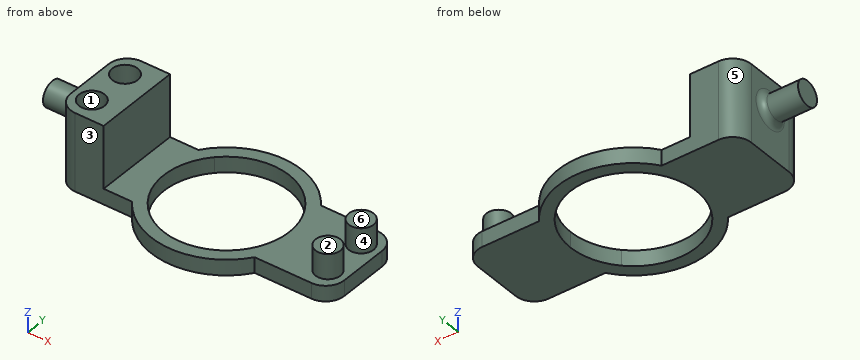
from build123d import *

# Parameters (mm, degrees)
EXTRUDE_1_DEPTH     = 2.5
FILLET_1_R          = 3
EXTRUDE_START       = 10
EXTRUDE_2_DEPTH     = 10
SKETCH_3_R          = 2
EXTRUDE_3_DEPTH     = 6
SKETCH_5_R          = 2
EXTRUDE_4_DEPTH     = 4
SKETCH_6_R          = 2.05
CUT_EXTRUDE_1_DEPTH = 4
FILLET_2_R          = 1


with BuildPart() as part:
    # 草图1 → 凸台-拉伸1 (new body)
    with BuildSketch(Plane.XY):
        with BuildLine():
            ThreePointArc((9.86965045, 7), (0, 12.1), (-9.86965045, 7))
            Line((-9.86965045, 7), (-7.28079666, 7))
            ThreePointArc((-7.28079666, 7), (0, 10.1), (7.28079666, 7))
            Line((7.28079666, 7), (9.86965045, 7))
        make_face()
        with BuildLine():
            Line((-22, 7), (-22, -7))
            Line((-22, -7), (-9.86965045, -7))
            ThreePointArc((-9.86965045, -7), (-12.1, 0), (-9.86965045, 7))
            Line((-9.86965045, 7), (-22, 7))
        make_face()
        with BuildLine():
            ThreePointArc((12.1, 0), (11.528936864, -3.673365593), (9.86965045, -7))
            Line((9.86965045, -7), (22, -7))
            Line((22, -7), (22, 7))
            Line((22, 7), (9.86965045, 7))
            ThreePointArc((9.86965045, 7), (11.528936864, 3.673365593), (12.1, 0))
        make_face()
        with BuildLine():
            Line((-7.28079666, -7), (-9.86965045, -7))
            ThreePointArc((-9.86965045, -7), (0, -12.1), (9.86965045, -7))
            Line((9.86965045, -7), (7.28079666, -7))
            ThreePointArc((7.28079666, -7), (0, -10.1), (-7.28079666, -7))
        make_face()
        with BuildLine():
            ThreePointArc((-9.86965045, 7), (-12.1, 0), (-9.86965045, -7))
            Line((-9.86965045, -7), (-7.28079666, -7))
            ThreePointArc((-7.28079666, -7), (-10.1, 0), (-7.28079666, 7))
            Line((-7.28079666, 7), (-9.86965045, 7))
        make_face()
        with BuildLine():
            Line((7.28079666, -7), (9.86965045, -7))
            ThreePointArc((9.86965045, -7), (11.528936864, -3.673365593), (12.1, 0))
            ThreePointArc((12.1, 0), (11.528936864, 3.673365593), (9.86965045, 7))
            Line((9.86965045, 7), (7.28079666, 7))
            ThreePointArc((7.28079666, 7), (9.368725801, 3.773191867), (10.1, 0))
            ThreePointArc((10.1, 0), (9.368725801, -3.773191867), (7.28079666, -7))
        make_face()
        with BuildLine():
            ThreePointArc((-9.86965045, 7), (-12.1, 0), (-9.86965045, -7))
            Line((-9.86965045, -7), (-7.28079666, -7))
            ThreePointArc((-7.28079666, -7), (-10.1, 0), (-7.28079666, 7))
            Line((-7.28079666, 7), (-9.86965045, 7))
        make_face()
        with BuildLine():
            Line((7.28079666, -7), (9.86965045, -7))
            ThreePointArc((9.86965045, -7), (11.528936864, -3.673365593), (12.1, 0))
            ThreePointArc((12.1, 0), (11.528936864, 3.673365593), (9.86965045, 7))
            Line((9.86965045, 7), (7.28079666, 7))
            ThreePointArc((7.28079666, 7), (9.368725801, 3.773191867), (10.1, 0))
            ThreePointArc((10.1, 0), (9.368725801, -3.773191867), (7.28079666, -7))
        make_face()
    extrude(amount=EXTRUDE_1_DEPTH)

    # 圆角1
    fillet_1_edges = [part.edges().sort_by_distance(p)[0] for p in [
        (22, 7, 1.25),
        (22, -7, 1.25),
        (-22, -7, 1.25),
        (-22, 7, 1.25),
    ]]
    fillet(fillet_1_edges, radius=FILLET_1_R)

    # 草图2 → 凸台-拉伸2 (add)
    with BuildSketch(Plane.XY.offset(2.5).offset(EXTRUDE_START)):
        with BuildLine():
            Line((-14.434825225, -7), (-14.434825225, 7))
            Line((-14.434825225, 7), (-19, 7))
            ThreePointArc((-19, 7), (-21.121320344, 6.121320344), (-22, 4))
            Line((-22, 4), (-22, -4))
            ThreePointArc((-22, -4), (-21.121320344, -6.121320344), (-19, -7))
            Line((-19, -7), (-14.434825225, -7))
        make_face()
    extrude(amount=-EXTRUDE_2_DEPTH)

    # 草图3 → 凸台-拉伸3 (add)
    with BuildSketch(Plane.ZY.offset(22)):
        with Locations(Location((7.5, 0, 0), (0, 0, 270))):
            Circle(SKETCH_3_R)
    extrude(amount=EXTRUDE_3_DEPTH)

    # 草图5 → 凸台-拉伸4 (add)
    with BuildSketch(Plane.XY.offset(2.5)):
        with Locations(Location((19, -3.5, 0), (0, 0, 180))):
            Circle(SKETCH_5_R)
        with Locations(Location((19, 3.5, 0), (0, 0, 180))):
            Circle(SKETCH_5_R)
    extrude(amount=EXTRUDE_4_DEPTH)

    # 草图6 → 切除-拉伸1 (cut)
    with BuildSketch(Plane.XY.offset(12.5)):
        with Locations((-19, 3.5)):
            Circle(SKETCH_6_R)
        with Locations((-19, -3.5)):
            Circle(SKETCH_6_R)
    extrude(amount=-CUT_EXTRUDE_1_DEPTH, mode=Mode.SUBTRACT)

    # 圆角2
    fillet_2_edges = [part.edges().sort_by_distance(p)[0] for p in [
        (-22, 2, 7.5),
    ]]
    fillet(fillet_2_edges, radius=FILLET_2_R)


solid = part.part
Verification items for the finished model (mm, model axes). Face numbers are marked on the shaded views. A direction names the side the tool comes from. Coordinates: 2 decimals unless noted, no trailing zeros. Order: outer loops, then holes, each group sorted by start corner. A loop starts at its lowest first (then second) coordinate and runs counter-clockwise, first axis right, second up. Notation, with made-up numbers: (71, 1.5) -> (93, 1.5) arc R24 cw to (93, 33.5) -> close; hole circle Ø10 at (6.25, -16.5). An arc over 180 degrees is marked (long way). Put each result on its own line as item: value. Start each with the question number.
1. Mould release check, pull along X, two halves, no side actions. Record for the marked faces 4, 5 and 6: released by +X, released by -X, zero draft, split by the parting line, or undercut.
2. Material ranges on L1, parallel to Y at x = -19, z = 10.1; L2, parallel to X at y = 0.5, z = 3.5; L3, parallel to Z at x = -14, y = 3.25, recorded low to high. Write a range as [from, to].
3. Go/stop test with flat-tipped pins: pin 1 Ø8 at (x, y) = (9.5, -4) entering from +Z; pin 2 Ø1.2 at (x, y) = (19, -3.5) entering from +Z; pin 3 Ø5 at (y, z) = (-2.5, 7) entering from +X. Record where each tip stops, or that it passes through.
4. Access from +Z, -Z, +X, -X, +Y, -Y to the whole of each face (thin tool, end or side, straight path). Record for the marked faces 1, 2 and 3.
5. Cross-section at C-C, the plane x = -5. Record the boundary of the cut face in (y, z), then the cut area to 3 significant figures.
6. Cross-section at B-B, the plane z = 1.5. Record the boundary of the cut face in (x, y), then the cut area to 3 significant figures.
7. Cross-section at D-D, the plane z = 7.5. Record the boundary of the cut face in (x, y).
8. Cross-section at A-A, the plane y = 3.5. Record the boundary of the cut face in (x, z).
Computed:
1. face 4: undercut
1. face 5: released by -X
1. face 6: zero draft
2. L1: [-7, -5.55], [-1.45, 1.45], [5.55, 7]
2. L2: [-22, -14.43]
2. L3: [0, 2.5]
3. pin 1: z = 2.5
3. pin 2: z = 6.5
3. pin 3: x = 21
4. face 1: +Z
4. face 2: +Z, +X, +Y, -Y
4. face 3: +Z, -Z, -X, -Y
5. outline: (-11.02, 0) -> (-8.78, 0) -> (-8.78, 2.5) -> (-11.02, 2.5) -> close; (8.78, 0) -> (11.02, 0) -> (11.02, 2.5) -> (8.78, 2.5) -> close
5. area: 11.2 mm2
6. outline: (-22, -4) arc R3 ccw to (-19, -7) -> (-9.87, -7) arc R12.1 ccw to (9.87, -7) -> (19, -7) arc R3 ccw to (22, -4) -> (22, 4) arc R3 ccw to (19, 7) -> (9.87, 7) arc R12.1 ccw to (-9.87, 7) -> (-19, 7) arc R3 ccw to (-22, 4) -> close; hole circle Ø20.2 at (0, 0)
6. area: 429 mm2
7. outline: (-28, -2) -> (-23, -2) arc R1 cw to (-22, -3) -> (-22, -4) arc R3 ccw to (-19, -7) -> (-14.43, -7) -> (-14.43, 7) -> (-19, 7) arc R3 ccw to (-22, 4) -> (-22, 3) arc R1 cw to (-23, 2) -> (-28, 2) -> close
8. outline: (-22, 0) -> (-9.47, 0) -> (-9.47, 2.5) -> (-14.43, 2.5) -> (-14.43, 12.5) -> (-16.95, 12.5) -> (-16.95, 8.5) -> (-21.05, 8.5) -> (-21.05, 12.5) -> (-22, 12.5) -> close; (9.47, 0) -> (22, 0) -> (22, 2.5) -> (21, 2.5) -> (21, 6.5) -> (17, 6.5) -> (17, 2.5) -> (9.47, 2.5) -> close
